from build123d import *

# Parameters (mm, degrees)
F1_DEPTH  = 13
F3_DEPTH  = 12
F5_DEPTH  = 8.8
F6_R      = 4.25
F7_DEPTH  = 13
F9_R      = 10
F9_R_2    = 4.25
F10_DEPTH = 2
F11_SIZE2 = 6
F11_SIZE  = 2


with BuildPart() as f1:
    # F0 (on Top) → F1 (new body)
    with BuildSketch(Plane.XY):
        Polygon((-17, -10), (17, -10), (34.1558913715, -6), (34.1558913715, 6), (17, 10), (-17, 10), (-38.0029598341, 6), (-38.0029598341, -6), align=None)
    extrude(amount=F1_DEPTH)

    # F2 (on face) → F3 (join)
    with BuildSketch(Plane.XY.offset(13)):
        with BuildLine():
            ThreePointArc((0, -10), (7.0710678119, -7.0710678119), (10, 0))
            ThreePointArc((10, 0), (7.0710677987, 7.0710678251), (-3.73e-08, 10))
            ThreePointArc((-3.73e-08, 10), (-10, -1.87e-08), (0, -10))
        make_face()
    extrude(amount=F3_DEPTH)

    # F4 (on face) → F5 (cut)
    with BuildSketch(Plane.XY.offset(25)):
        Polygon((-3.8105117767, -6.6), (3.8105117767, -6.6), (7.6210235533, 0), (3.8105117767, 6.6), (-3.8105117767, 6.6), (-7.6210235533, 0), align=None)
    extrude(amount=-F5_DEPTH, mode=Mode.SUBTRACT)

    # F6 (on face) → F7 (cut)
    with BuildSketch(Plane.XY.offset(16.2)):
        Circle(F6_R)
    extrude(amount=-F7_DEPTH, mode=Mode.SUBTRACT)

    # F9 (on offset) → F10 (join)
    with BuildSketch(Plane.XY.offset(23)):
        Circle(F9_R)
        Circle(F9_R_2, mode=Mode.SUBTRACT)
    extrude(amount=F10_DEPTH)

    # F11
    f11_edges = [f1.edges().sort_by_distance(p)[0] for p in [
        (0, -10, 0),
        (-27.50148, -8, 0),
        (-38.00296, 0, 0),
        (25.577946, -8, 0),
        (34.155891, 0, 0),
        (25.577946, 8, 0),
        (0, 10, 0),
        (-27.50148, 8, 0),
    ]]
    f11_side = f1.faces().sort_by_distance((-1.644994, 0, 0))[0]
    chamfer(f11_edges, length=F11_SIZE, length2=F11_SIZE2, reference=f11_side)


solid = f1.part
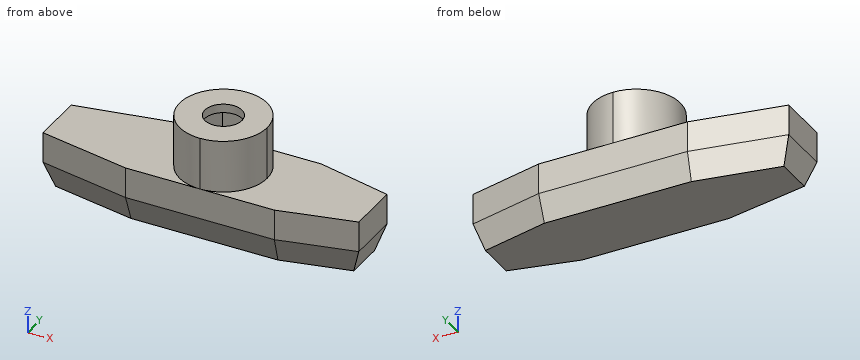
Source: CAD feature listing. Evaluate the final solid. Frame: model axes, mm. Give positions to 0.01 mm unless a question says otherwise; leave off trailing zeros. Write each loop counter-clockwise with the first axis right and the second up, starting at its lowest first coordinate (ties: lowest second). Pieces come first, ordered by that corner, then holes. Notation, with made-up numbers: (42.25, -21) -> (46.25, -21) arc R13 cw to (46.25, 2) -> close; hole circle Ø6 at (-15, -16). An arc over 180 degrees is marked (long way). Write item = value, one per line.
Q1. Line query: line 1 (Y direction, x = 0, z = 11.75); line 2 (Z direction, x = -5, y = -0.5); line 3 (Z direction, x = -19, y = 4.25). Output: solid intervals per line, ascending. Write a range as from..to.
Here are the results:
line_1 = -10..-4.25, 4.25..10
line_2 = 0..16.2, 23..25
line_3 = 0..13
Q2. Cut plane B-B on x = -6.5. Return loops of the section in (y, z).
Here are the results:
outline = (-10, 6) -> (-8, 0) -> (8, 0) -> (10, 6) -> (10, 13) -> (7.6, 13) -> (7.6, 25) -> (-7.6, 25) -> (-7.6, 13) -> (-10, 13) -> close; hole (-1.94, 16.2) -> (1.94, 16.2) -> (1.94, 23) -> (-1.94, 23) -> close
Q3. Cut plane A-A on z = 22.25. Return loops of the section in (x, y), then the cut area to 3 significant figures.
Here are the results:
outline = circle Ø20 at (0, 0); hole (-7.62, 0) -> (-3.81, -6.6) -> (3.81, -6.6) -> (7.62, 0) -> (3.81, 6.6) -> (-3.81, 6.6) -> close
area = 163 mm²
Q4. First-contact query: pin 1 (1.5 mm diameter, centred on y = -4.5, z = 17.5, fed in from -X); pin 2 (6 mm diameter, centred on y = -7, z = 18.5, fed in from -X); pin 3 (4 mm diameter, centred on x = -0.5, y = 1.5, fed in from +Z). Flat tips, straight axial feed; report the tip coordinate or a pass-through.
Here are the results:
pin_1 = -9.27
pin_2 = -9.17
pin_3 = 3.2
Q5. Cut plane D-D on x = 1.5. Return loops of the section in (y, z), then the cut area to 3 significant figures.
Here are the results:
outline = (-10, 6) -> (-8, 0) -> (8, 0) -> (10, 6) -> (10, 13) -> (9.89, 13) -> (9.89, 25) -> (3.98, 25) -> (3.98, 23) -> (6.6, 23) -> (6.6, 16.2) -> (3.98, 16.2) -> (3.98, 3.2) -> (-3.98, 3.2) -> (-3.98, 16.2) -> (-6.6, 16.2) -> (-6.6, 23) -> (-3.98, 23) -> (-3.98, 25) -> (-9.89, 25) -> (-9.89, 13) -> (-10, 13) -> close
area = 276 mm²
Q6. Cut plane C-C on z = 11.5. Return loops of the section in (x, y), then the cut area to 3 significant figures.
Here are the results:
outline = (-38, -6) -> (-17, -10) -> (17, -10) -> (34.16, -6) -> (34.16, 6) -> (17, 10) -> (-17, 10) -> (-38, 6) -> close; hole circle Ø8.5 at (0, 0)
area = 1,230 mm²
